from build123d import *

# Parameters (mm, degrees)
SKETCH_1_W          = 50
SKETCH_1_H          = 10
EXTRUDE_1_DEPTH     = 5
SKETCH_2_R          = 1.5
CUT_EXTRUDE_1_DEPTH = 26.980762114
SKETCH_3_W          = 15
SKETCH_3_H          = 2.5
CUT_EXTRUDE_2_DEPTH = 28.386127875


with BuildPart() as part:
    # 草图1 → 凸台-拉伸1 (new body)
    with BuildSketch(Plane(origin=(0, 0, 0), x_dir=(1, 0, 0), z_dir=(0, 1, 0))):
        Rectangle(SKETCH_1_W, SKETCH_1_H)
    extrude(amount=EXTRUDE_1_DEPTH)

    # 草图2 → 切除-拉伸1 (cut, through all)
    with BuildSketch(Plane(origin=(0, 5, 0), x_dir=(1, 0, 0), z_dir=(0, 1, 0))):
        with Locations(Location((22, 2, 0), (0, 0, 270))):
            Circle(SKETCH_2_R)
        with Locations(Location((19, -2, 0), (0, 0, 270))):
            Circle(SKETCH_2_R)
    extrude(amount=-CUT_EXTRUDE_1_DEPTH, mode=Mode.SUBTRACT)

    # 草图3 → 切除-拉伸2 (cut, through all)
    with BuildSketch(Plane.XY.offset(5)):
        with Locations((-17.5, 3.75)):
            Rectangle(SKETCH_3_W, SKETCH_3_H)
    extrude(amount=-CUT_EXTRUDE_2_DEPTH, mode=Mode.SUBTRACT)


solid = part.part
Geometry: final body of the model. Coordinates: model frame, mm. A direction names the side the tool comes from. Coordinates: 2 decimals unless noted, no trailing zeros. Order: outer loops, then holes, each group sorted by start corner. A loop starts at its lowest first (then second) coordinate and runs counter-clockwise, first axis right, second up.
1) Section C-C (y = 3.45). Return loops of the section in (x, z), then the cut area to 3 significant figures.
Result sheet:
outline: (-10, -5) - (25, -5) - (25, 5) - (-10, 5) - close; hole circle Ø3 at (19, 2); hole circle Ø3 at (22, -2)
area: 336 mm2
2) Section A-A (x = 19). Return loops of the section in (y, z).
Result sheet:
outline: (0, -5) - (5, -5) - (5, 0.5) - (0, 0.5) - close; (0, 3.5) - (5, 3.5) - (5, 5) - (0, 5) - close
3) Set-up query: faces 1 (the flat face through (-18, 2.5, 0)), 2 (the flat face through (0, 0, 0)). Return all of +Z, -Z, +X, -X, +Y, -Y with unobstructed straight access to the full face (end or side cutting, diameter ignored); none if empty.
Result sheet:
face 1: +Z, -Z, -X, +Y
face 2: +Z, -Z, +X, -X, -Y
4) Ray query, probe 1 along X at (y, z) = (1.55, -2); probe 2 along X at (y, z) = (3.35, -2); probe 3 along Y at (x, z) = (-20, -2.5). Return the intervals inside material, ascending.
Result sheet:
probe 1: x = -25 to 20.5, 23.5 to 25
probe 2: x = -10 to 20.5, 23.5 to 25
probe 3: y = 0 to 2.5
5) Section B-B (z = -2). Return loops of the section in (x, y).
Result sheet:
outline: (-25, 0) - (20.5, 0) - (20.5, 5) - (-10, 5) - (-10, 2.5) - (-25, 2.5) - close; (23.5, 0) - (25, 0) - (25, 5) - (23.5, 5) - close
6) Section D-D (z = -4.5). Return loops of the section in (x, y).
Result sheet:
outline: (-25, 0) - (25, 0) - (25, 5) - (-10, 5) - (-10, 2.5) - (-25, 2.5) - close
7) First-contact query: P1, Ø3, axis at x = -20, z = 0.5, coming from the +Y side; P2, Ø1.8, axis at x = 22, z = -2, coming from the -Y side. Flat tips, straight axial feed; report the tip coordinate or a pass-through.
Result sheet:
P1: stops at y = 2.5
P2: passes through
8) Draft query along X for faces 3 (the cylindrical face through (23.265, 2.535, -1.194)), 4 (the flat face through (-10, 4, 0)), 5 (the flat face through (5, 2, -5)). Return one class per face: released by +X, released by -X, zero draft, split by the parting line, or undercut.
Result sheet:
face 3: undercut
face 4: released by -X
face 5: zero draft
